The listing builds one solid part. Answer for the finished solid, in the listing's coordinates (mm). A direction names the side the tool comes from. Give positions to 0.01 mm unless a question says otherwise; leave off trailing zeros. Write each loop counter-clockwise with the first axis right and the second up, starting at its lowest first coordinate (ties: lowest second). Pieces come first, ordered by that corner, then holes. Notation, with made-up numbers: M 5.5,20 L 32.5,20 A27 cw 32.5,49 Z; hole C 55.25,-22 d5. An arc over 180 degrees is marked long. Answer as a JSON object with one key per item and string values.
```python
from build123d import *

# Parameters (mm, degrees)
SKETCH1_R               = 16
SKETCH1_R_2             = 1.5
SKETCH1_R_3             = 3
BOSS_EXTRUDE1_DEPTH     = 4
SKETCH2_R               = 6.5
SKETCH2_R_2             = 3
BOSS_EXTRUDE2_DEPTH     = 10
FILLET1_R               = 1
CUT_EXTRUDE1_DEPTH      = 27.608269391
CUT_EXTRUDE1_DEPTH_BACK = 27.608269391
SKETCH3_R               = 1.25
CHAMFER1_SIZE           = 0.5


with BuildPart() as part:
    # Sketch1 → Boss-Extrude1 (new body)
    with BuildSketch(Plane(origin=(0, 0, 0), x_dir=(1, 0, 0), z_dir=(0, 1, 0))):
        with Locations(Location((0, 0, 0), (0, 0, 270))):
            Circle(SKETCH1_R)
        with Locations(Location((0, 11.691342951, 0), (0, 0, 270))):
            Circle(SKETCH1_R_2, mode=Mode.SUBTRACT)
        with Locations(Location((10.125, 5.845671476, 0), (0, 0, 270))):
            Circle(SKETCH1_R_2, mode=Mode.SUBTRACT)
        with Locations(Location((10.125, -5.845671476, 0), (0, 0, 270))):
            Circle(SKETCH1_R_2, mode=Mode.SUBTRACT)
        with Locations(Location((0, -11.691342951, 0), (0, 0, 270))):
            Circle(SKETCH1_R_2, mode=Mode.SUBTRACT)
        with Locations(Location((-10.125, -5.845671476, 0), (0, 0, 270))):
            Circle(SKETCH1_R_2, mode=Mode.SUBTRACT)
        with Locations(Location((-10.125, 5.845671476, 0), (0, 0, 270))):
            Circle(SKETCH1_R_2, mode=Mode.SUBTRACT)
        with Locations(Location((0, 0, 0), (0, 0, 270))):
            Circle(SKETCH1_R_3, mode=Mode.SUBTRACT)
    extrude(amount=BOSS_EXTRUDE1_DEPTH)

    # Sketch2 → Boss-Extrude2 (add)
    with BuildSketch(Plane(origin=(0, 4, 0), x_dir=(1, 0, 0), z_dir=(0, 1, 0))):
        with Locations(Location((0, 0, 0), (0, 0, 270))):
            Circle(SKETCH2_R)
        with Locations(Location((0, 0, 0), (0, 0, 270))):
            Circle(SKETCH2_R_2, mode=Mode.SUBTRACT)
    extrude(amount=BOSS_EXTRUDE2_DEPTH)

    # Fillet1
    fillet1_edges = [part.edges().sort_by_distance(p)[0] for p in [
        (0, 4, -6.5),
    ]]
    fillet(fillet1_edges, radius=FILLET1_R)

    # Sketch3 → Cut-Extrude1 (cut, two sides: drawn at the far end of the back side and taken through both)
    with BuildSketch(Plane.XY.offset(-CUT_EXTRUDE1_DEPTH_BACK)):
        with Locations((0, 9)):
            Circle(SKETCH3_R)
    extrude(amount=CUT_EXTRUDE1_DEPTH + CUT_EXTRUDE1_DEPTH_BACK, mode=Mode.SUBTRACT)

    # Chamfer1
    chamfer1_edges = [part.edges().sort_by_distance(p)[0] for p in [
        (0, 0, -16),
        (0, 14, -6.5),
        (0, 4, -16),
    ]]
    chamfer(chamfer1_edges, length=CHAMFER1_SIZE)


solid = part.part
```
1. A cutting plane is placed at A-A, the plane z = 0. Give the vertices of the cut face in (x, y), plus the area to 3 significant figures.
Verdict:
{"outline": "M -16,0.5 L -15.5,0 L -3,0 L -3,14 L -6,14 L -6.5,13.5 L -6.5,5 A1 cw -7.5,4 L -15.5,4 L -16,3.5 Z; M 3,0 L 15.5,0 L 16,0.5 L 16,3.5 L 15.5,4 L 7.5,4 A1 cw 6.5,5 L 6.5,13.5 L 6,14 L 3,14 Z", "area": "174 mm2"}
2. For faces 1 (the cylindrical face through (-11.59, 1.97, -6.17)), 2 (the cylindrical face through (1.95, 9.19, 6.2)), determine the directions among +Z, -Z, +X, -X, +Y, -Y from which every point of the face is accessible in a straight line to the end or side of a thin tool.
Verdict:
{"face 1": "+Y, -Y", "face 2": "+Y"}
3. The mould has two halves that part along Y. Classify faces 3 (the flat face through (4, 4, 7)), 4 (the cylindrical face through (1.19, 9.38, -4.64)), 5 (the cylindrical face through (-1.15, 6.9, 2.77)): released by +Y, released by -Y, zero draft, split by the parting line, or undercut.
Verdict:
{"face 3": "released by +Y", "face 4": "undercut", "face 5": "zero draft"}
4. A cutting plane is placed at B-B, the plane y = 9. Give the vertices of the cut face in (x, z).
Verdict:
{"outline": "M -1.25,-6.38 L -1.25,-2.73 A3 cw -1.25,2.73 L -1.25,6.38 A6.5 ccw Z; M 1.25,-6.38 A6.5 ccw 1.25,6.38 L 1.25,2.73 A3 cw 1.25,-2.73 Z"}
5. Consider line 1 along X through (y, z) = (3.25, 6); line 2 along Z through (x, y) = (0.5, 3.5); line 3 along X through (y, z) = (2, 5.5). Determine where each line is inside the solid, lowest interval first.
Verdict:
{"line 1": "x = -14.83 to -11.62, -8.63 to 8.63, 11.62 to 14.83", "line 2": "z = -15.99 to -13.11, -10.28 to -2.96, 2.96 to 10.28, 13.11 to 15.99", "line 3": "x = -15.02 to -11.58, -8.67 to 8.67, 11.58 to 15.02"}
6. Flat-ended cylindrical pins translate along their axes: pin 1 (1 mm diameter, centred on y = 10, z = -2, fed in from +X); pin 2 (5 mm diameter, centred on x = 2, z = -10.5, fed in from +Y); pin 3 (2 mm diameter, centred on x = -4.5, y = 9.5, fed in from -Z). Find the tip coordinate at first contact, or state that the pin passes through.
Verdict:
{"pin 1": "stops at x = 6.32", "pin 2": "stops at y = 4", "pin 3": "stops at z = -5.48"}
7. A cutting plane is placed at C-C, the plane x = 0. Count the separate pieces of the cut face and the enclosed holes in it, plus the area to 3 significant figures.
Verdict:
{"separate pieces": "6", "enclosed holes": "0", "area": "132 mm2"}
